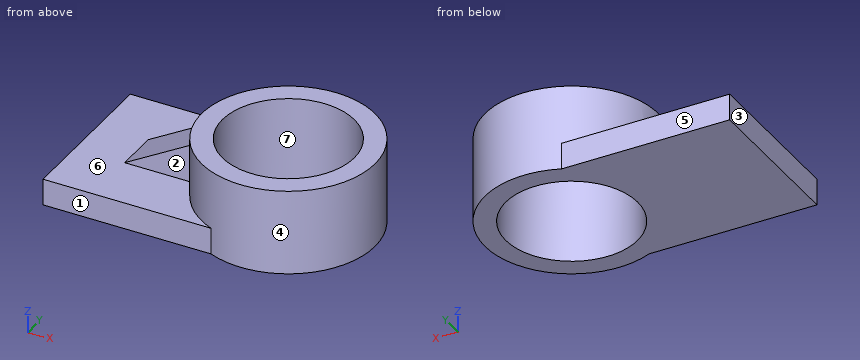
from build123d import *

# Parameters (mm, degrees)
F0_W     = 193.0230408907
F0_H     = 152.3501798511
F2_DEPTH = 25.4
F3_DEPTH = 82.042
F4_R     = 82.7208063485
F4_R_2   = 62.9840996432
F5_DEPTH = 81.788
F7_DEPTH = 62.992
F9_DEPTH = 46.228


with BuildPart() as f2:
    # F0 (on Top) → F2 (new body)
    with BuildSketch(Plane.XY):
        with Locations((-20.3011333942, 0.0200085342)):
            Rectangle(F0_W, F0_H)
    extrude(amount=F2_DEPTH)

    # F1 (on face) → F3 (cut)
    with BuildSketch(Plane.XY):
        with BuildLine():
            Line((76.2103870511, -63.3074275445), (76.2103870511, 63.3074275445))
            ThreePointArc((76.2103870511, 63.3074275445), (12.8221735358, 0), (76.2103870511, -63.3074275445))
        make_face()
    extrude(amount=F3_DEPTH, mode=Mode.SUBTRACT)

    # F4 (on Top) → F5 (join)
    with BuildSketch(Plane.XY):
        with Locations((75.9201049805, 0)):
            Circle(F4_R)
        with Locations((75.9201049805, 0)):
            Circle(F4_R_2, mode=Mode.SUBTRACT)
    extrude(amount=F5_DEPTH)

    # F6 (on face) → F7 (join)
    with BuildSketch(Plane(origin=(0, 0, 0), x_dir=(1, 0, 0), z_dir=(0, 0, -1))):
        Polygon((8.5411956534, -20.6989627331), (8.5411956534, 0), (8.5411956534, 20.5139704049), (-69.3054571748, 20.5139704049), (-69.3054571748, -20.6989627331), align=None)
    extrude(amount=-F7_DEPTH)

    # F8 (on face) → F9 (cut)
    with BuildSketch(Plane.XZ.offset(20.5139704049)):
        Polygon((-69.3054571748, 25.4), (-4.2167081654, 62.992), (-69.3054571748, 62.992), align=None)
    extrude(amount=-F9_DEPTH, mode=Mode.SUBTRACT)


solid = f2.part
Here's how the part is built. I have some questions about the finished solid (model axes, mm). Face numbers are marked on the shaded views. A direction names the side the tool comes from. Coordinates: 2 decimals unless noted, no trailing zeros. Order: outer loops, then holes, each group sorted by start corner. A loop starts at its lowest first (then second) coordinate and runs counter-clockwise, first axis right, second up. Notation, with made-up numbers: (52, 87.25) - (80, 87.25) arc R26 ccw to (80, 105.25) - close; hole circle Ø9 at (63, 76.25). An arc over 180 degrees is marked (long way). Use CSV: the item, a comma, the result in double quotes. Start each with the question number.
1. Suppose I cut it at B-B on x = 50.5. List the corners of the cut face in (y, z) for me, then the cut area to 3 significant figures.
2. Suppose I cut it at D-D on x = -49. List the corners of the cut face in (y, z) for me, then the cut area to 3 significant figures.
3. I'm going to push flat-ended pins straight in: pin 1 (4 mm diameter, centred on y = -13, z = 41.5, fed in from +X); pin 2 (1 mm diameter, centred on y = 11, z = 60.5, fed in from +X); pin 3 (8 mm diameter, centred on y = 55, z = 17.5, fed in from +X). Where does each tip first touch, or does it pass through?
4. Please list where these lines run through material, in increasing order: line 1 (Y direction, x = -33, z = 11); line 2 (Z direction, x = 3, y = -49.5); line 3 (X direction, y = -53, z = 6). Write a range as from..to.
5. For the marked faces 1, 2 and 3, which set-ups out of +Z, -Z, +X, -X, +Y, -Y let a thin tool reach every point of the face, with its end or its side?
6. Suppose I cut it at A-A on y = 0. List the corners of the cut face in (x, z) for me, then the cut area to 3 significant figures.
7. If we mould it in two halves opening along Y, with no side actions, what happens to the marked faces 4, 5, 6 and 7? For each: +Y half, -Y half, draft (parallel to the pull), parting line (faces both ways), or undercut.
8. Suppose I cut it at C-C on z = 22. List the corners of the cut face in (x, y) for me, then the cut area to 3 significant figures.
Output:
1,outline,"(-78.72, 0) - (-57.63, 0) - (-57.63, 81.79) - (-78.72, 81.79) - close; (57.63, 0) - (78.72, 0) - (78.72, 81.79) - (57.63, 81.79) - close"
1,area,"3,450 mm2"
2,outline,"(-76.16, 0) - (76.2, 0) - (76.2, 25.4) - (20.7, 25.4) - (20.7, 37.13) - (-20.51, 37.13) - (-20.51, 25.4) - (-76.16, 25.4) - close"
2,area,"4,350 mm2"
3,pin 1,"stops at x = 157.91"
3,pin 2,"stops at x = 157.97"
3,pin 3,"stops at x = 141.05"
4,line 1,"y = -76.16..76.2"
4,line 2,"z = 0..25.4"
4,line 3,"x = -116.81..41.89, 109.95..139.43"
5,face 1,"+Z, -Z, -X, -Y"
5,face 2,"+Z, -X, -Y"
5,face 3,"+Z, -Z, -X, +Y, -Y"
6,outline,"(-116.81, 0) - (12.94, 0) - (12.94, 81.79) - (-6.8, 81.79) - (-6.8, 62.99) - (-4.22, 62.99) - (-69.31, 25.4) - (-116.81, 25.4) - close; (138.9, 0) - (158.64, 0) - (158.64, 81.79) - (138.9, 81.79) - close"
6,area,"7,150 mm2"
7,face 4,"parting line"
7,face 5,"+Y half"
7,face 6,"draft"
7,face 7,"undercut"
8,outline,"(-116.81, -76.16) - (43.62, -76.16) arc R82.72 ccw (long way) to (43.72, 76.2) - (-116.81, 76.2) - close; hole circle Ø125.97 at (75.92, 0)"
8,area,"27,900 mm2"
